from build123d import *

# Parameters (mm, degrees)
BOSS_EXTRUDE2_DEPTH     = 279.4
CUT_EXTRUDE1_DEPTH      = 279.4
FILLET1_R               = 2.54
SKETCH7_W               = 192.0875
SKETCH7_H               = 254
CUT_EXTRUDE2_DEPTH      = 44.45
SKETCH8_W               = 6.173248721
SKETCH8_H               = 35.639061591
BOSS_EXTRUDE3_DEPTH     = 258.064
CUT_EXTRUDE3_DEPTH      = 260.35
CUT_EXTRUDE3_DEPTH_BACK = 6.35
CUT_EXTRUDE4_DEPTH      = 260.35
CUT_EXTRUDE4_DEPTH_BACK = 6.35
BOSS_EXTRUDE4_DEPTH     = 254
SKETCH18_R              = 3.175
CUT_EXTRUDE5_DEPTH      = 71.12


with BuildPart() as part:
    # CrossSection → Boss-Extrude2 (new body)
    with BuildSketch(Plane.XY):
        with BuildLine():
            Line((108.74375, 11.322324676), (108.74375, -50.8))
            Line((108.74375, -50.8), (-108.74375, -50.8))
            Line((-108.74375, -50.8), (-108.74375, 11.322324676))
            ThreePointArc((-108.74375, 11.322324676), (0, 0), (108.74375, 11.322324676))
        make_face()
    extrude(amount=BOSS_EXTRUDE2_DEPTH)

    # Sketch4 → Cut-Extrude1 (cut)
    with BuildSketch(Plane(origin=(0, 0, 0), x_dir=(-1, 0, 0), z_dir=(0, 0, -1))):
        with BuildLine():
            ThreePointArc((0, -50.8), (-54.665798723, -47.96178867), (-108.74375, -39.477675324))
            Line((-108.74375, -39.477675324), (-108.74375, -50.8))
            Line((-108.74375, -50.8), (0, -50.8))
        make_face()
        with BuildLine():
            ThreePointArc((108.74375, -39.477675324), (54.665798723, -47.96178867), (0, -50.8))
            Line((0, -50.8), (108.74375, -50.8))
            Line((108.74375, -50.8), (108.74375, -39.477675324))
        make_face()
    extrude(amount=-CUT_EXTRUDE1_DEPTH, mode=Mode.SUBTRACT)

    # Fillet1
    fillet1_edges = [part.edges().sort_by_distance(p)[0] for p in [
        (108.74375, -39.477675324, 139.7),
        (-108.74375, -39.477675324, 139.7),
    ]]
    fillet(fillet1_edges, radius=FILLET1_R)

    # Sketch7 → Cut-Extrude2 (cut)
    with BuildSketch(Plane(origin=(0, -50.8, 0), x_dir=(1, 0, 0), z_dir=(0, 1, 0))):
        with Locations((0, -139.7)):
            Rectangle(SKETCH7_W, SKETCH7_H)
    extrude(amount=CUT_EXTRUDE2_DEPTH, mode=Mode.SUBTRACT)

    # Sketch8 → Boss-Extrude3 (add)
    with BuildSketch(Plane.XY.offset(12.7)):
        with Locations((3.086624361, -24.169530796)):
            Rectangle(SKETCH8_W, SKETCH8_H)
        with Locations((-3.086624361, -24.169530796)):
            Rectangle(SKETCH8_W, SKETCH8_H)
    extrude(amount=BOSS_EXTRUDE3_DEPTH)

    # Sketch13 → Cut-Extrude3 (cut, two sides: drawn at the far end of the back side and taken through both)
    with BuildSketch(Plane.XY.offset(12.7).offset(-CUT_EXTRUDE3_DEPTH_BACK)):
        with BuildLine():
            ThreePointArc((-96.04375, -40.123592373), (-48.223527841, -46.727181022), (0, -48.934530782))
            Line((0, -48.934530782), (0, -43.854530782))
            ThreePointArc((0, -43.854530782), (-48.223527841, -41.647181022), (-96.04375, -35.043592373))
            Line((-96.04375, -35.043592373), (-96.04375, -37.583592373))
            Line((-96.04375, -37.583592373), (-96.04375, -40.123592373))
        make_face()
        with BuildLine():
            Line((0, -43.854530782), (0, -48.934530782))
            ThreePointArc((0, -48.934530782), (48.223527841, -46.727181022), (96.04375, -40.123592373))
            Line((96.04375, -40.123592373), (96.04375, -37.583592373))
            Line((96.04375, -37.583592373), (96.04375, -35.043592373))
            ThreePointArc((96.04375, -35.043592373), (48.223527841, -41.647181022), (0, -43.854530782))
        make_face()
    extrude(amount=CUT_EXTRUDE3_DEPTH + CUT_EXTRUDE3_DEPTH_BACK, mode=Mode.SUBTRACT)

    # Sketch14 → Cut-Extrude4 (cut, two sides: drawn at the far end of the back side and taken through both)
    with BuildSketch(Plane(origin=(0, 0, 266.7), x_dir=(-1, 0, 0), z_dir=(0, 0, -1)).offset(-CUT_EXTRUDE4_DEPTH_BACK)):
        with BuildLine():
            Line((96.04375, -35.043592373), (96.04375, -40.123592373))
            ThreePointArc((96.04375, -40.123592373), (-28.026510339, -48.189989717), (-150.541934286, -27.012946445))
            Line((-150.541934286, -27.012946445), (-150.541934286, -21.932946445))
            ThreePointArc((-150.541934286, -21.932946445), (-28.026510339, -43.109989717), (96.04375, -35.043592373))
        make_face()
    extrude(amount=CUT_EXTRUDE4_DEPTH + CUT_EXTRUDE4_DEPTH_BACK, mode=Mode.SUBTRACT)

    # Sketch15 → Boss-Extrude4 (add)
    with BuildSketch(Plane(origin=(0, 0, 266.7), x_dir=(-1, 0, 0), z_dir=(0, 0, -1))):
        with BuildLine():
            Line((6.173248721, -43.818432493), (6.173248721, -41.989061591))
            Line((6.173248721, -41.989061591), (-6.173248721, -41.989061591))
            Line((-6.173248721, -41.989061591), (-6.173248721, -43.818432493))
            ThreePointArc((-6.173248721, -43.818432493), (0, -43.854530782), (6.173248721, -43.818432493))
        make_face()
    extrude(amount=BOSS_EXTRUDE4_DEPTH)

    # Sketch18 → Cut-Extrude5 (cut)
    with BuildSketch(Plane(origin=(0, -50.8, 0), x_dir=(1, 0, 0), z_dir=(0, 1, 0))):
        with Locations(Location((101.380501252, -209.55, 0), (0, 0, 90))):
            Circle(SKETCH18_R)
        with Locations(Location((101.380501252, -69.85, 0), (0, 0, 90))):
            Circle(SKETCH18_R)
    extrude(amount=CUT_EXTRUDE5_DEPTH, mode=Mode.SUBTRACT)


solid = part.part
Geometry check sheet. Reference: the model listing, model coordinates, mm. A direction names the side the tool comes from. Round coordinates to 2 decimals unless told otherwise and drop trailing zeros. Loops run counter-clockwise (first coordinate to the right, second up) from the corner with the lowest first, then second, coordinate; pieces in that order, holes last.
Item 1: Cross-section at A-A on z = 182. Record the boundary of the cut face in (x, y), then the cut area to 3 significant figures.
Item 2: Gauge pin test, flat ends, axial feed: pin 1 (1.5 mm diameter, centred on x = -76.5, z = 105, fed in from -Y); pin 2 (7.5 mm diameter, centred on x = 101.38, z = 209.55, fed in from +Y); pin 3 (4 mm diameter, centred on x = 101.38, z = 69.85, fed in from +Y). Record the tip position at first contact, or that the pin passes through.
Item 3: Cross-section at D-D on z = 69.85. Record the boundary of the cut face in (x, y).
Item 4: Access from +Z, -Z, +X, -X, +Y, -Y to the whole of each face (thin tool, end or side, straight path). Record for faces 1 (the flat face through (-52, -25, 266.7)), 2 (the flat face through (6, -45, 273.05)), 3 (the cylindrical face through (-1.533, 0.002, 137.744)).
Item 5: Cross-section at C-C on x = -55.5. Record the boundary of the cut face in (y, z), then the cut area to 3 significant figures.
Item 6: Mould release check, pull along X, two halves, no side actions. Record for faces 4 (the flat face through (2, -19, 0)), 5 (the flat face through (108.744, -7, 138)), 6 (the flat face through (-52, -25, 12.7)), 7 (the flat face through (-108.744, -13, 138)): pulls with the +X half, pulls with the -X half, needs draft (parallel to the pull), parting line crosses it, or undercut.
Item 7: Cross-section at B-B on y = -23. Count the separate pieces of the cut face and the enclosed holes in it, then the cut area to 3 significant figures.
Item 8: Thickness scan on line 1 (X direction, y = -24, z = 165); line 2 (X direction, y = -8, z = 69.85); line 3 (Z direction, x = -25.5, y = -35). Record the ranges inside material, lowest first.
Answer sheet:
1. outline: (-108.74, -37.41) arc R2.54 ccw to (-106.72, -39.9) arc R527.87 ccw to (-96.04, -41.99) - (-96.04, -6.35) - (-6.17, -6.35) - (-6.17, -43.82) arc R527.87 ccw to (6.17, -43.82) - (6.17, -6.35) - (96.04, -6.35) - (96.04, -35.04) arc R527.87 ccw to (108.74, -32.53) - (108.74, 11.32) arc R527.87 cw to (-108.74, 11.32) - close; (96.04, -41.99) arc R527.87 ccw to (106.72, -39.9) arc R2.54 ccw to (108.74, -37.61) arc R527.87 cw to (96.04, -40.12) - close
1. area: 3,470 mm2
2. pin 1: stops at y = -6.35
2. pin 2: stops at y = 10.57
2. pin 3: passes through
3. outline: (-108.74, -37.41) arc R2.54 ccw to (-106.72, -39.9) arc R527.87 ccw to (-96.04, -41.99) - (-96.04, -6.35) - (-6.17, -6.35) - (-6.17, -43.82) arc R527.87 ccw to (6.17, -43.82) - (6.17, -6.35) - (96.04, -6.35) - (96.04, -35.04) arc R527.87 ccw to (98.21, -34.64) - (98.21, 9.22) arc R527.87 cw to (-108.74, 11.32) - close; (96.04, -41.99) arc R527.87 ccw to (98.21, -41.58) - (98.21, -39.72) arc R527.87 cw to (96.04, -40.12) - close; (104.56, -40.34) arc R527.87 ccw to (106.72, -39.9) arc R2.54 ccw to (108.74, -37.61) arc R527.87 cw to (104.56, -38.48) - close; (104.56, -33.4) arc R527.87 ccw to (108.74, -32.53) - (108.74, 11.32) arc R527.87 cw to (104.56, 10.46) - close
4. face 1: -Y
4. face 2: none
4. face 3: +Z, -Z, +Y
5. outline: (-47.87, 0) - (2.93, 0) - (2.93, 279.4) - (-47.87, 279.4) - (-47.87, 266.7) - (-46.01, 266.7) - (-46.01, 273.05) - (-40.93, 273.05) - (-40.93, 266.7) - (-6.35, 266.7) - (-6.35, 12.7) - (-40.93, 12.7) - (-40.93, 6.35) - (-46.01, 6.35) - (-46.01, 12.7) - (-47.87, 12.7) - close
5. area: 3,580 mm2
6. face 4: needs draft
6. face 5: pulls with the +X half
6. face 6: undercut
6. face 7: pulls with the -X half
7. separate pieces: 1
7. enclosed holes: 4
7. area: 15,000 mm2
8. line 1: x = -108.74 to -96.04, -6.17 to 6.17, 96.04 to 108.74
8. line 2: x = -108.74 to -96.04, -6.17 to 6.17, 96.04 to 98.21, 104.56 to 108.74
8. line 3: z = 0 to 12.7, 266.7 to 279.4
